```python
from build123d import *

# Parameters (mm, degrees)
SKETCH1_R           = 4
SKETCH1_R_2         = 1.5
BOSS_EXTRUDE1_DEPTH = 3


with BuildPart() as part:
    # Sketch1 → Boss-Extrude1 (new body)
    with BuildSketch(Plane.XY):
        with BuildLine():
            Line((-70, 6), (70, 6))
            ThreePointArc((70, 6), (72.121320344, 5.121320344), (73, 3))
            Line((73, 3), (73, -3))
            ThreePointArc((73, -3), (72.121320344, -5.121320344), (70, -6))
            Line((70, -6), (-70, -6))
            ThreePointArc((-70, -6), (-72.121320344, -5.121320344), (-73, -3))
            Line((-73, -3), (-73, 3))
            ThreePointArc((-73, 3), (-72.121320344, 5.121320344), (-70, 6))
        make_face()
        with Locations((-66, 0)):
            Circle(SKETCH1_R, mode=Mode.SUBTRACT)
        with Locations((66, 0)):
            Circle(SKETCH1_R, mode=Mode.SUBTRACT)
        with Locations((-55, 0)):
            Circle(SKETCH1_R_2, mode=Mode.SUBTRACT)
        with Locations((55, 0)):
            Circle(SKETCH1_R_2, mode=Mode.SUBTRACT)
        with BuildLine():
            Line((-46, 1.5), (-4, 1.5))
            ThreePointArc((-4, 1.5), (-3.010050506, 1.089949494), (-2.6, 0.1))
            Line((-2.6, 0.1), (-2.6, -0.1))
            ThreePointArc((-2.6, -0.1), (-3.010050506, -1.089949494), (-4, -1.5))
            Line((-4, -1.5), (-46, -1.5))
            ThreePointArc((-46, -1.5), (-46.989949494, -1.089949494), (-47.4, -0.1))
            Line((-47.4, -0.1), (-47.4, 0.1))
            ThreePointArc((-47.4, 0.1), (-46.989949494, 1.089949494), (-46, 1.5))
        make_face(mode=Mode.SUBTRACT)
        with BuildLine():
            Line((4, 1.5), (46, 1.5))
            ThreePointArc((46, 1.5), (46.989949494, 1.089949494), (47.4, 0.1))
            Line((47.4, 0.1), (47.4, -0.1))
            ThreePointArc((47.4, -0.1), (46.989949494, -1.089949494), (46, -1.5))
            Line((46, -1.5), (4, -1.5))
            ThreePointArc((4, -1.5), (3.010050506, -1.089949494), (2.6, -0.1))
            Line((2.6, -0.1), (2.6, 0.1))
            ThreePointArc((2.6, 0.1), (3.010050506, 1.089949494), (4, 1.5))
        make_face(mode=Mode.SUBTRACT)
    extrude(amount=BOSS_EXTRUDE1_DEPTH)


solid = part.part
```
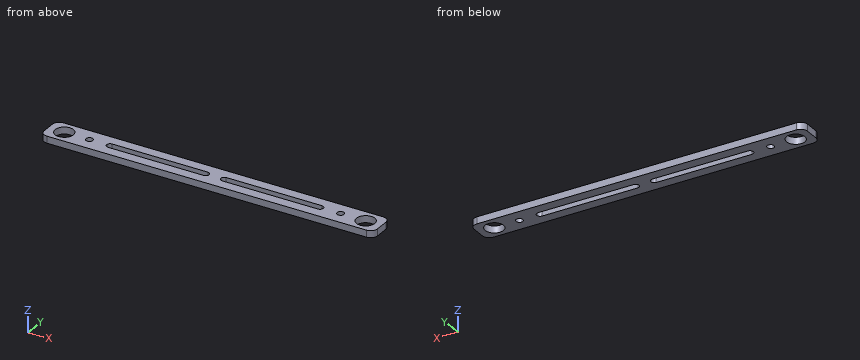
Geometry: final body of the model. Coordinates: model frame, mm. Round coordinates to 2 decimals unless told otherwise and drop trailing zeros. Order: outer loops, then holes, each group sorted by start corner. A loop starts at its lowest first (then second) coordinate and runs counter-clockwise, first axis right, second up. Notation, with made-up numbers: (-37, -37) -> (-20, -37) arc R10 ccw to (-20, -24) -> close; hole circle Ø7 at (8, 88.5). An arc over 180 degrees is marked (long way). Write each question's results on one line, items separated by ' | '.
Q1. Ray query, line 1 along Y through (x, z) = (18.5, 0.25); line 2 along Y through (x, z) = (-66, 1.65); line 3 along X through (y, z) = (2.75, 2.75). Return the intervals inside material, ascending.
Response values:
line 1: -6 to -1.5, 1.5 to 6 | line 2: -6 to -4, 4 to 6 | line 3: -73 to -68.9, -63.1 to 63.1, 68.9 to 73
Q2. Section query B-B (z = 1.75). Output: boundary loops of the cut face in (x, y), and give its area (3 significant figures).
Response values:
outline: (-73, -3) arc R3 ccw to (-70, -6) -> (70, -6) arc R3 ccw to (73, -3) -> (73, 3) arc R3 ccw to (70, 6) -> (-70, 6) arc R3 ccw to (-73, 3) -> close; hole circle Ø8 at (-66, 0); hole circle Ø3 at (-55, 0); hole (-47.4, -0.1) arc R1.4 ccw to (-46, -1.5) -> (-4, -1.5) arc R1.4 ccw to (-2.6, -0.1) -> (-2.6, 0.1) arc R1.4 ccw to (-4, 1.5) -> (-46, 1.5) arc R1.4 ccw to (-47.4, 0.1) -> close; hole (2.6, -0.1) arc R1.4 ccw to (4, -1.5) -> (46, -1.5) arc R1.4 ccw to (47.4, -0.1) -> (47.4, 0.1) arc R1.4 ccw to (46, 1.5) -> (4, 1.5) arc R1.4 ccw to (2.6, 0.1) -> close; hole circle Ø3 at (55, 0); hole circle Ø8 at (66, 0) | area: 1,360 mm²
Q3. Section query A-A (x = -55). Output: boundary loops of the cut face in (y, z), and give its area (3 significant figures).
Response values:
outline: (-6, 0) -> (-1.5, 0) -> (-1.5, 3) -> (-6, 3) -> close; (1.5, 0) -> (6, 0) -> (6, 3) -> (1.5, 3) -> close | area: 27.0 mm²
